For this review, take the finished solid that the model builds, in its own axes (mm). Face numbers are marked on the shaded views. A direction names the side the tool comes from. Round coordinates to 2 decimals unless told otherwise and drop trailing zeros. Order: outer loops, then holes, each group sorted by start corner. A loop starts at its lowest first (then second) coordinate and runs counter-clockwise, first axis right, second up. Notation, with made-up numbers: M -32,-1.75 L -18,-1.75 A27 ccw -18,24.25 Z; hole C -2.75,76.25 d7. An arc over 180 degrees is marked long. Use a Markdown table: item, result.
from build123d import *

# Parameters (mm, degrees)
F0_W     = 83
F0_H     = 103
F1_DEPTH = 30
F2_W     = 80
F2_H     = 100
F3_DEPTH = 27


with BuildPart() as f1:
    # F0 (on Top) → F1 (new body)
    with BuildSketch(Plane.XY):
        Rectangle(F0_W, F0_H)
    extrude(amount=-F1_DEPTH)

    # F2 (on Top) → F3 (cut)
    with BuildSketch(Plane.XY):
        Rectangle(F2_W, F2_H)
    extrude(amount=-F3_DEPTH, mode=Mode.SUBTRACT)


solid = f1.part
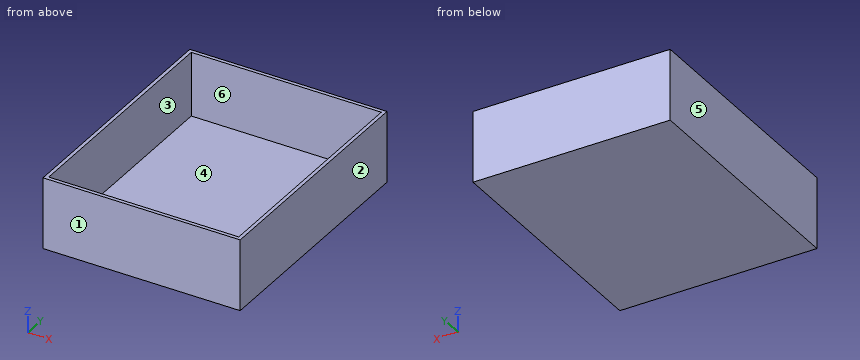
Q1. Add section B-B (y = 26.5). Write out the cut boundary in (x, z), then the cut area to 3 significant figures.
Determined:
| item | result |
|---|---|
| outline | M -41.5,-30 L 41.5,-30 L 41.5,0 L 40,0 L 40,-27 L -40,-27 L -40,0 L -41.5,0 Z |
| area | 330 mm^2 |
Q2. Draft analysis for pull direction X (two halves, no side actions). For the marked faces 1, 2, 3 and 4, state which applies: pulls with the +X half, pulls with the -X half, needs draft (parallel to the pull), parting line crosses it, or undercut.
Determined:
| item | result |
|---|---|
| face 1 | needs draft |
| face 2 | pulls with the +X half |
| face 3 | undercut |
| face 4 | undercut |
Q3. Machinability: for the marked faces 5 and 6, which of the approach directions +Z, -Z, +X, -X, +Y, -Y give a long, thin tool a straight path to every point of the face, cutting with its end or side? Answer none if there is none.
Determined:
| item | result |
|---|---|
| face 5 | +Z, -Z, -X, +Y, -Y |
| face 6 | +Z |
Q4. Clearance check with a flat-ended pin moving along its axis: pin 1 (2 mm diameter, centred on x = 24.5, y = 39, fed in from +Z). State where the tip first meets the part, or that it passes through.
Determined:
| item | result |
|---|---|
| pin 1 | stops at z = -27 |
Q5. Add section C-C (x = 34). Write out the cut boundary in (y, z), then the cut area to 3 significant figures.
Determined:
| item | result |
|---|---|
| outline | M -51.5,-30 L 51.5,-30 L 51.5,0 L 50,0 L 50,-27 L -50,-27 L -50,0 L -51.5,0 Z |
| area | 390 mm^2 |
Q6. Add section A-A (z = -9.25). Write out the cut boundary in (x, y), then the cut area to 3 significant figures.
Determined:
| item | result |
|---|---|
| outline | M -41.5,-51.5 L 41.5,-51.5 L 41.5,51.5 L -41.5,51.5 Z; hole M -40,-50 L 40,-50 L 40,50 L -40,50 Z |
| area | 549 mm^2 |
Q7. Wall thickness on line 1 along X through (y, z) = (6, -1.5); line 2 along Y through (x, z) = (-17.5, -11.75); line 3 along Z through (x, y) = (37, -28.5): over which ranges is each line inside the solid? List them lowest first. Write a range as [from, to].
Determined:
| item | result |
|---|---|
| line 1 | x = [-41.5, -40], [40, 41.5] |
| line 2 | y = [-51.5, -50], [50, 51.5] |
| line 3 | z = [-30, -27] |
